from build123d import *

# Parameters (mm, degrees)
F1_DEPTH = 1000
F2_R     = 11.5
F3_DEPTH = 175
F6_R     = 11.5
F7_DEPTH = 25


with BuildPart() as f1:
    # F0 (on Front) → F1 (new body)
    with BuildSketch(Plane.XZ):
        with BuildLine():
            Line((50, 75), (-38, 75))
            ThreePointArc((-38, 75), (-46.485281, 71.485281), (-50, 63))
            Line((-50, 63), (-50, -63))
            ThreePointArc((-50, -63), (-46.485281, -71.485281), (-38, -75))
            Line((-38, -75), (50, -75))
            Line((50, -75), (50, -69))
            Line((50, -69), (-39, -69))
            ThreePointArc((-39, -69), (-42.535534, -67.535534), (-44, -64))
            Line((-44, -64), (-44, 64))
            ThreePointArc((-44, 64), (-42.535534, 67.535534), (-39, 69))
            Line((-39, 69), (50, 69))
            Line((50, 69), (50, 75))
        make_face()
    extrude(amount=F1_DEPTH)

    # F2 (on face) → F3 (cut)
    with BuildSketch(Plane.XY.offset(75)):
        with Locations((10, -60)):
            Circle(F2_R)
        with Locations((10, -940)):
            Circle(F2_R)
    extrude(amount=-F3_DEPTH, mode=Mode.SUBTRACT)

    # F6 (on face) → F7 (cut)
    with BuildSketch(Plane.XY.offset(75)):
        with Locations((0, -497.356147)):
            Circle(F6_R)
    extrude(amount=-F7_DEPTH, mode=Mode.SUBTRACT)


with BuildPart() as f4_1:
    # F4: copy of F1
    add(f1.part.moved(Location((300, 0, 0))))


solid = f1.part
Part model, mm, in its own coordinate system. A direction names the side the tool comes from. Give positions to 0.01 mm unless a question says otherwise; leave off trailing zeros. Loops run counter-clockwise (first coordinate to the right, second up) from the corner with the lowest first, then second, coordinate; pieces in that order, holes last. Notation, with made-up numbers: (80.5, 28) -> (104.5, 28) arc R26 cw to (104.5, 42) -> close; hole circle Ø6 at (8, 33.25). An arc over 180 degrees is marked (long way). Write each question's results on one line, items separated by ' | '. Start each with the question number.
Q1. Band-saw the part on C-C on z = 30.5. List the corners of the cut face in (x, y).
Q2. Band-saw the part on B-B on y = -363.5. List the corners of the cut face in (x, z).
Q3. Which spindle directions (+Z, -Z, +X, -X, +Y, -Y) get a long thin tool onto all of the face, cutting with end or side? Do faces 4 (the face through (-1.497, -485.954, 72.042)), 5 (the face through (-44, -493, -1)), 6 (the face through (7.507, -71.227, 72.042)). Say none if no direction does.
Q4. Pull direction X, two halves, no side cores. Call faces 1 (the face through (16.18, -930.3, -71.96)), 2 (the face through (-50, -493, 1)), 3 (the face through (-45, -1000, 0)): +X half, -X half, draft (parallel to the pull), parting line (faces both ways), or undercut.
Q5. Pin check, flat tips, straight feed: P1, Ø1.5, axis at y = -826.5, z = 46, coming from the +X side; P2, Ø14, axis at x = 10, y = -60, coming from the -Z side. Stop position of each tip, or through.
Q6. Band-saw the part on A-A on y = -60. List the corners of the cut face in (x, z), plus the area to 3 significant figures.
Q7. Wall check: L1, parallel to Y at x = 10, z = -72.2; L2, parallel to Z at x = -3, y = -300.5; L3, parallel to Y at x = 10, z = 73.65. Give the ranges that are in metal, low to high.
Results are:
1) outline: (-50, -1000) -> (-44, -1000) -> (-44, 0) -> (-50, 0) -> close
2) outline: (-50, -63) arc R12 ccw to (-38, -75) -> (50, -75) -> (50, -69) -> (-39, -69) arc R5 cw to (-44, -64) -> (-44, 64) arc R5 cw to (-39, 69) -> (50, 69) -> (50, 75) -> (-38, 75) arc R12 ccw to (-50, 63) -> close
3) face 4: +Z | face 5: +X, +Y, -Y | face 6: +Z, -Z
4) face 1: undercut | face 2: -X half | face 3: draft
5) P1: stops at x = -44 | P2: passes through
6) outline: (-50, -63) arc R12 ccw to (-38, -75) -> (-1.5, -75) -> (-1.5, -69) -> (-39, -69) arc R5 cw to (-44, -64) -> (-44, 64) arc R5 cw to (-39, 69) -> (-1.5, 69) -> (-1.5, 75) -> (-38, 75) arc R12 ccw to (-50, 63) -> close; (21.5, -75) -> (50, -75) -> (50, -69) -> (21.5, -69) -> close; (21.5, 69) -> (50, 69) -> (50, 75) -> (21.5, 75) -> close | area: 1,700 mm²
7) L1: y = -1000 to -951.5, -928.5 to -71.5, -48.5 to 0 | L2: z = -75 to -69, 69 to 75 | L3: y = -1000 to -951.5, -928.5 to -503.04, -491.68 to -71.5, -48.5 to 0
